For this review, take the finished solid that the model builds, in its own axes (mm). A direction names the side the tool comes from. Round coordinates to 2 decimals unless told otherwise and drop trailing zeros. Order: outer loops, then holes, each group sorted by start corner. A loop starts at its lowest first (then second) coordinate and runs counter-clockwise, first axis right, second up. Notation, with made-up numbers: (87, 41) -> (119, 41) arc R28 cw to (119, 78) -> close; hole circle Ø10 at (-7.75, 8.5). An arc over 180 degrees is marked (long way). Use a Markdown table: item, result. Add a question column.
1) Consider section C-C (y = 31). State the section outline as (x, z) points.
2) Consider section B-B (x = 73.5). State the section outline as (y, z) points.
3) Machinability: for faces 1 (the face through (2, 280, 2)), 2 (the face through (131, 5, 2)), which of the approach directions +Z, -Z, +X, -X, +Y, -Y give a long, thin tool a straight path to every point of the face, cutting with its end or side? Answer none if there is none.
4) Consider section A-A (z = 3.45). State the section outline as (x, y) points, plus the area to 3 significant figures.
5) Draft analysis for pull direction Y (two halves, no side actions). For faces 3 (the face through (43.855, 67.158, 2.465)), 4 (the face through (91, 0, 2)), 5 (the face through (0, 138, 2)), 6 (the face through (91.28, 144.42, 2.46)), state which applies: pulls with the +Y half, pulls with the -Y half, needs draft (parallel to the pull), parting line crosses it, or undercut.
6) Wall thickness on line 1 along Y through (x, z) = (30, 1.9); line 2 along Y through (x, z) = (81, 1.1); line 3 along X through (y, z) = (81, 1.4): over which ranges is each line inside the solid? List them lowest first. Write a range as [from, to].
7) Consider section D-D (y = 188.5). State the section outline as (x, z) points, plus the area to 3 significant figures.
8) Clearance check with flat-ended pins moving along their axes: P1, Ø2, axis at x = 49, z = 1.5, coming from the +Y side; P2, Ø1.5, axis at y = 58.5, z = 3.5, coming from the +X side; P3, Ø2.5, axis at y = 177.5, z = 3.5, coming from the +X side. State where each tip first meets the part, or that it passes through.
```python
from build123d import *

# Parameters (mm, degrees)
BOSS_EXTRUDE1_DEPTH = 5


with BuildPart() as part:
    # Sketch1 → Boss-Extrude1 (new body)
    with BuildSketch(Plane.XY):
        Polygon((0, 0), (0, 280), (5, 280), (180, 5), (180, 0), align=None)
        Polygon((89.757735174, 5), (174.073452359, 5), (5, 270.686853707), (5, 136.845365827), align=None, mode=Mode.SUBTRACT)
        Polygon((5, 5), (5, 127.599078617), (83.813693397, 5), align=None, mode=Mode.SUBTRACT)
    extrude(amount=BOSS_EXTRUDE1_DEPTH)


solid = part.part
```
Results list:
| question | item | result |
|---|---|---|
| 1 | outline | (0, 0) -> (5, 0) -> (5, 5) -> (0, 5) -> close; (67.1, 0) -> (73.04, 0) -> (73.04, 5) -> (67.1, 5) -> close; (157.53, 0) -> (163.45, 0) -> (163.45, 5) -> (157.53, 5) -> close |
| 2 | outline | (0, 0) -> (5, 0) -> (5, 5) -> (0, 5) -> close; (21.04, 0) -> (30.29, 0) -> (30.29, 5) -> (21.04, 5) -> close; (163.04, 0) -> (172.36, 0) -> (172.36, 5) -> (163.04, 5) -> close |
| 3 | face 1 | +Z, -Z, +X, -X, +Y |
| 3 | face 2 | +Z, -Z |
| 4 | outline | (0, 0) -> (180, 0) -> (180, 5) -> (5, 280) -> (0, 280) -> close; hole (5, 5) -> (83.81, 5) -> (5, 127.6) -> close; hole (5, 136.85) -> (89.76, 5) -> (174.07, 5) -> (5, 270.69) -> close |
| 4 | area | 4,630 mm2 |
| 5 | face 3 | undercut |
| 5 | face 4 | pulls with the -Y half |
| 5 | face 5 | needs draft |
| 5 | face 6 | pulls with the +Y half |
| 6 | line 1 | [0, 5], [88.71, 97.96], [231.4, 240.71] |
| 6 | line 2 | [0, 5], [9.38, 18.62], [151.26, 160.57] |
| 6 | line 3 | [0, 5], [34.96, 40.9], [125.71, 131.64] |
| 7 | outline | (0, 0) -> (5, 0) -> (5, 5) -> (0, 5) -> close; (57.3, 0) -> (63.23, 0) -> (63.23, 5) -> (57.3, 5) -> close |
| 7 | area | 54.6 mm2 |
| 8 | P1 | y = 212.43 |
| 8 | P2 | x = 146.43 |
| 8 | P3 | x = 71.02 |
